Can you work these out from the model? Positions are in its coordinate system, mm. Face numbers are marked on the shaded views. Coordinates: 2 decimals unless noted, no trailing zeros. Loops run counter-clockwise (first coordinate to the right, second up) from the corner with the lowest first, then second, coordinate; pieces in that order, holes last. Notation, with made-up numbers: (68, 76) -> (90, 76) arc R19 cw to (90, 82) -> close; hole circle Ø3 at (18, 42). An arc over 180 degrees is marked (long way). Use one line per item in the form item = value. Start each with the question number.
(1) Thinking about a two-plate mould opening in X: for the marked faces 1, 2, 3 and 4, which applies, released by +X, released by -X, zero draft, split by the parting line, or undercut?
(2) Imagine slicing it at A-A (x = -9). List the corners of the cut face in (y, z) for me.
(3) Imagine slicing it at C-C (y = 9.25). List the corners of the cut face in (x, z) for me, plus the area to 3 significant figures.
(4) Imagine slicing it at D-D (x = 10). List the corners of the cut face in (y, z) for me, plus the area to 3 significant figures.
(5) I need wall thicknesses on line 1 (X direction, y = 6.75, z = 0); line 2 (Y direction, x = -5, z = -3.5); line 3 (Z direction, x = 9, y = 2.05). Which ranges of each line are inside material? Lowest first, please. Write a range as [from, to].
(6) Imagine slicing it at B-B (z = -1.5). State how many separate pieces and enclosed holes the cut face has, plus the area to 3 significant figures.
(7) I'm going to push flat-ended pins straight in: pin 1 (4.5 mm diameter, centred on x = 0, z = 0, fed in from +Y); pin 2 (1.5 mm diameter, centred on y = 1.5, z = 2, fed in from -X); pin 3 (5 mm diameter, centred on y = 6.5, z = 0, fed in from +X); pin 4 (1 mm diameter, centred on x = 2, y = 10, fed in from -Z). Where does each tip first touch, or does it pass through?
```python
from build123d import *

# Parameters (mm, degrees)
EXTRUDE_1_DEPTH     = 3.5
SKETCH_2_R          = 5
EXTRUDE_2_DEPTH     = 8.5
SKETCH_3_R          = 2.5
CUT_EXTRUDE_1_DEPTH = 19.034688797
SKETCH_4_R          = 1.75
CUT_EXTRUDE_2_DEPTH = 16.921683328
CHAMFER_1_SIZE      = 0.5


with BuildPart() as part:
    # 草图1 → 凸台-拉伸1 (new body)
    with BuildSketch(Plane(origin=(0, 0, 0), x_dir=(1, 0, 0), z_dir=(0, 1, 0))):
        with BuildLine():
            ThreePointArc((-11.456439237, 5), (-12.236328912, 2.553870546), (-12.5, 0))
            Line((-12.5, 0), (12.5, 0))
            ThreePointArc((12.5, 0), (12.236328912, 2.553870546), (11.456439237, 5))
            Line((11.456439237, 5), (-11.456439237, 5))
        make_face()
        with BuildLine():
            Line((12.5, 0), (-12.5, 0))
            ThreePointArc((-12.5, 0), (-12.236328912, -2.553870546), (-11.456439237, -5))
            Line((-11.456439237, -5), (11.456439237, -5))
            ThreePointArc((11.456439237, -5), (12.236328912, -2.553870546), (12.5, 0))
        make_face()
    extrude(amount=EXTRUDE_1_DEPTH)

    # 草图2 → 凸台-拉伸2 (add)
    with BuildSketch(Plane(origin=(0, 3.5, 0), x_dir=(1, 0, 0), z_dir=(0, 1, 0))):
        with Locations(Location((0, 0, 0), (0, 0, 270))):
            Circle(SKETCH_2_R)
    extrude(amount=EXTRUDE_2_DEPTH)

    # 草图3 → 切除-拉伸1 (cut, through all)
    with BuildSketch(Plane(origin=(0, 12, 0), x_dir=(1, 0, 0), z_dir=(0, 1, 0))):
        with Locations(Location((0, 0, 0), (0, 0, 270))):
            Circle(SKETCH_3_R)
    extrude(amount=-CUT_EXTRUDE_1_DEPTH, mode=Mode.SUBTRACT)

    # 草图4 → 切除-拉伸2 (cut, through all)
    with BuildSketch(Plane(origin=(0, 3.5, 0), x_dir=(1, 0, 0), z_dir=(0, 1, 0))):
        with Locations(Location((-9, 0, 0), (0, 0, 270))):
            Circle(SKETCH_4_R)
        with Locations(Location((9, 0, 0), (0, 0, 90))):
            Circle(SKETCH_4_R)
    extrude(amount=-CUT_EXTRUDE_2_DEPTH, mode=Mode.SUBTRACT)

    # 倒角1
    chamfer_1_edges = [part.edges().sort_by_distance(p)[0] for p in [
        (0, 12, -5),
        (0, 12, -2.5),
    ]]
    chamfer(chamfer_1_edges, length=CHAMFER_1_SIZE)


solid = part.part
```
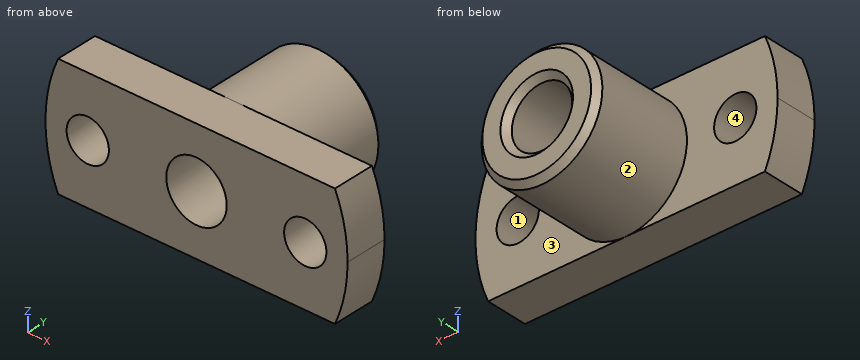
Worked out:
q1.face_1 = undercut
q1.face_2 = split by the parting line
q1.face_3 = zero draft
q1.face_4 = undercut
q2.outline = (0, -5) -> (3.5, -5) -> (3.5, -1.75) -> (0, -1.75) -> close; (0, 1.75) -> (3.5, 1.75) -> (3.5, 5) -> (0, 5) -> close
q3.outline = circle Ø10 at (0, 0); hole circle Ø5 at (0, 0)
q3.area = 58.9 mm2
q4.outline = (0, -5) -> (3.5, -5) -> (3.5, -1.44) -> (0, -1.44) -> close; (0, 1.44) -> (3.5, 1.44) -> (3.5, 5) -> (0, 5) -> close
q4.area = 24.9 mm2
q5.line_1 = [-5, -2.5], [2.5, 5]
q5.line_2 = [0, 3.5]
q5.line_3 = [-5, -1.75], [1.75, 5]
q6.separate_pieces = 4
q6.enclosed_holes = 0
q6.area = 107 mm2
q7.pin_1 = through
q7.pin_2 = -12.44
q7.pin_3 = 5
q7.pin_4 = -4.77
